Build history of the part. All positions in model axes, mm. Face numbers are marked on the shaded views. A direction names the side the tool comes from. Round coordinates to 2 decimals unless told otherwise and drop trailing zeros. Write each loop counter-clockwise with the first axis right and the second up, starting at its lowest first coordinate (ties: lowest second). Pieces come first, ordered by that corner, then holes.
from build123d import *

# Parameters (mm, degrees)
BOSS_EXTRUDE1_DEPTH      = 7
BOSS_EXTRUDE1_DEPTH_BACK = 7
SKETCH2_R                = 2.75
CUT_EXTRUDE1_DEPTH       = 3
SKETCH3_R                = 2.75
CUT_EXTRUDE2_DEPTH       = 3


with BuildPart() as part:
    # Sketch1 → Boss-Extrude1 (new, two sides: drawn at the far end of the back side and taken through both)
    with BuildSketch(Plane(origin=(0, 0, 0), x_dir=(0, 0, -1), z_dir=(1, 0, 0)).offset(-BOSS_EXTRUDE1_DEPTH_BACK)):
        Polygon((-20, 0), (0, 0), (0, 20), (-3, 20), (-3, 3), (-20, 3), align=None)
    extrude(amount=BOSS_EXTRUDE1_DEPTH + BOSS_EXTRUDE1_DEPTH_BACK)

    # Sketch2 → Cut-Extrude1 (cut)
    with BuildSketch(Plane.XY):
        with Locations((0, 10)):
            Circle(SKETCH2_R)
    extrude(amount=CUT_EXTRUDE1_DEPTH, mode=Mode.SUBTRACT)

    # Sketch3 → Cut-Extrude2 (cut)
    with BuildSketch(Plane(origin=(0, 0, 0), x_dir=(1, 0, 0), z_dir=(0, 1, 0))):
        with Locations(Location((0, -15, 0), (0, 0, 270))):
            Circle(SKETCH3_R)
    extrude(amount=CUT_EXTRUDE2_DEPTH, mode=Mode.SUBTRACT)


solid = part.part
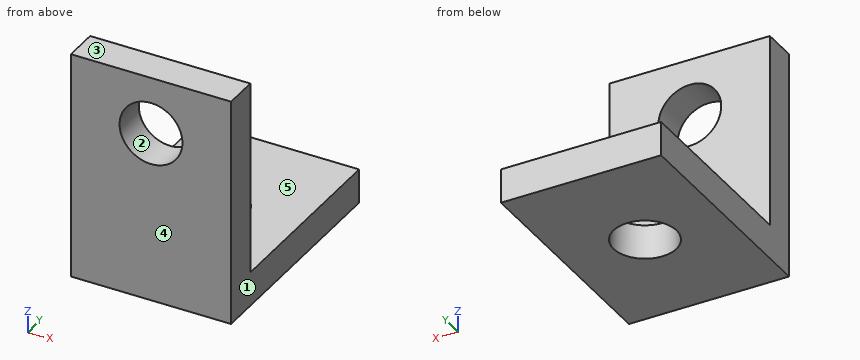
1) Which spindle directions (+Z, -Z, +X, -X, +Y, -Y) get a long thin tool onto all of the face, cutting with end or side? Do the marked faces 4 and 5. Say none if no direction does.
Results:
face 4: +Z, -Z, +X, -X, -Y
face 5: +Z, +X, -X, +Y
2) Slice it at A-A (z = 15). Write the cut outline in (x, y), plus the area to 3 significant figures.
Results:
outline: (-7, 0) - (-2.75, 0) - (-2.75, 3) - (-7, 3) - close; (2.75, 0) - (7, 0) - (7, 3) - (2.75, 3) - close
area: 25.5 mm2
3) Pin check, flat tips, straight feed: pin 1 Ø7 at (x, y) = (0, 10) entering from +Z; pin 2 Ø5 at (x, z) = (4.5, 13) entering from +Y; pin 3 Ø4 at (x, z) = (2, 16.5) entering from -Y. Stop position of each tip, or through.
Results:
pin 1: stops at z = 3
pin 2: stops at y = 3
pin 3: stops at y = 0
4) Slice it at C-C (x = 1). Write the cut outline in (y, z), plus the area to 3 significant figures.
Results:
outline: (0, 0) - (7.44, 0) - (7.44, 3) - (3, 3) - (3, 12.44) - (0, 12.44) - close; (0, 17.56) - (3, 17.56) - (3, 20) - (0, 20) - close; (12.56, 0) - (20, 0) - (20, 3) - (12.56, 3) - close
area: 80.3 mm2
5) Slice it at D-D (y = 1.5). Write the cut outline in (x, z).
Results:
outline: (-7, 0) - (7, 0) - (7, 20) - (-7, 20) - close; hole circle Ø5.5 at (0, 15)
6) Mould opens along Z. For the marked faces 1, 2 and 3 say: released by +Z, released by -Z, zero draft, split by the parting line, or undercut.
Results:
face 1: zero draft
face 2: undercut
face 3: released by +Z
7) Wall check: L1, parallel to Y at x = 0, z = 0.85; L2, parallel to Y at x = 3, z = 5.5; L3, parallel to X at y = 2.3, z = 15. Give the ranges that are in metal, low to high.
Results:
L1: y = 0 to 7.25, 12.75 to 20
L2: y = 0 to 3
L3: x = -7 to -2.75, 2.75 to 7
